Here's how the part is built. I have some questions about the finished solid (model axes, mm). Face numbers are marked on the shaded views. A direction names the side the tool comes from. Round coordinates to 2 decimals unless told otherwise and drop trailing zeros. Loops run counter-clockwise (first coordinate to the right, second up) from the corner with the lowest first, then second, coordinate; pieces in that order, holes last. Notation, with made-up numbers: M 0,85.5 L 42,85.5 A24 ccw 42,107.5 Z; hole C 38.25,-17 d2. An arc over 180 degrees is marked long. Answer as a JSON object with one key per item and string values.
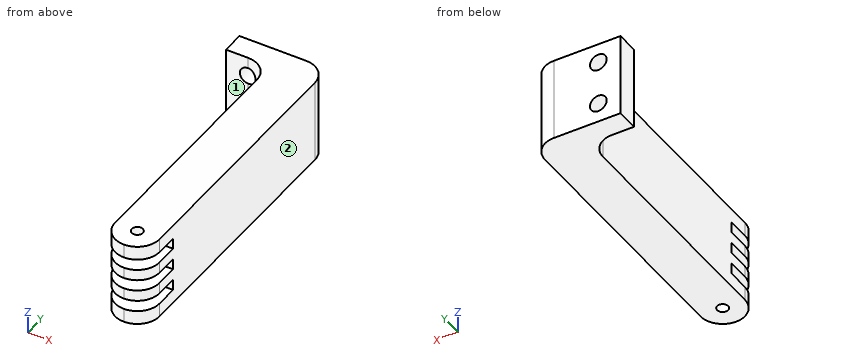
Autodesk Inventor part; units mm, degrees
ref_plane "YZ Plane" through (0, 0, 0) normal (1, 0, 0) x (0, 1, 0)
ref_plane "XZ Plane" through (0, 0, 0) normal (0, 1, 0) x (-1, 0, 0)
ref_plane "XY Plane" through (0, 0, 0) normal (0, 0, 1) x (1, 0, 0)
sketch "Sketch1" plane through (0, 0, 0) normal (0, 0, 1) x (1, 0, 0)
  line L0 (0, 0) -> (0, 50)
  line L1 (0, 50) -> (-8, 50)
  line L2 (0, 0) -> (8, 0)
  line L3 (8, 0) -> (8, 54)
  line L4 (8, 54) -> (-8, 54)
  line L5 (8, 54) -> (-8, 54)
  line L6 (-8, 54) -> (-8, 50)
  dimension "d0" = 50
  dimension "d3" = 8
  dimension "d7" = 54
  dimension "d28" = 16
extrude "Extrusion1" add sketch "Sketch1" along normal blind 15
sketch "Sketch2" plane through (-8, 54, 0) normal (0, 1, 0) x (1, 0, 0)
  line L0 (16, 0) -> (0, 0) construction
  line L1 (1.2766, 0) -> (1.2766, -15) construction
  line L2 (16, -15) -> (0, -15) construction
  line L3 (1.2766, 0) -> (1.2766, -2.75) construction
  line L4 (1.2766, -15) -> (1.2766, -12.25) construction
  line L5 (1.2766, 0) -> (1.2766, -3.5) construction
  line L6 (1.2766, -15) -> (1.2766, -11.5) construction
  line L7 (8, 0) -> (0, 0) construction
  line L8 (0, 0) -> (0, -15) construction
  line L9 (4, 0) -> (4, -15) construction
  line L10 (4, -15) -> (4, -11.5) construction
  line L11 (4, 0) -> (4, -3.5) construction
  circle A0 centre (4, -3.5) radius 1.5
  circle A1 centre (4, -11.5) radius 1.5
  dimension "d12" = 3.5
  dimension "d13" = 3.5
  dimension "d29" = 3.5
  dimension "d30" = 3.5
  dimension "d31" = 3
  dimension "d32" = 3
extrude "Extrusion2" cut sketch "Sketch2" against normal blind 8.75
sketch "Sketch3" plane through (8, 0, 0) normal (1, 0, 0) x (0, 0, -1)
  line L0 (0, 0) -> (-15, 0) construction
  line L1 (-7.5, 0) -> (-7.5, 8) construction
  line L2 (-7.5, 8) -> (-6.5, 8)
  line L3 (-6.5, 8) -> (-8.5, 8)
  line L4 (-8.5, 8) -> (-8.5, 0)
  line L5 (-6.5, 8) -> (-6.5, 0)
  line L6 (-6.5, 0) -> (-4.5, 0)
  line L7 (-4.5, 0) -> (-4.5, 8)
  line L8 (-4.5, 8) -> (-2.5, 8)
  line L9 (-2.5, 8) -> (-2.5, 0)
  line L10 (-8.5, 0) -> (-10.5, 0)
  line L11 (-10.5, 0) -> (-10.5, 8)
  line L12 (-10.5, 8) -> (-12.5, 8)
  line L13 (-12.5, 8) -> (-12.5, 0)
  line L14 (-2.5, 0) -> (0, 0)
  line L15 (-12.5, 0) -> (-15, 0)
  line L16 (-15, 0) -> (-15, 10)
  line L17 (-15, 50) -> (-15, 0)
  line L18 (-15, 10) -> (0, 10)
  line L19 (0, 50) -> (0, 0)
  line L20 (0, 0) -> (0, 10)
  line L21 (-15, 0) -> (0, 0)
  dimension "d18" = 8
  dimension "d19" = 1
  dimension "d20" = 2
  dimension "d21" = 2
  dimension "d22" = 2
  dimension "d23" = 2
  dimension "d24" = 2
  dimension "d25" = 10
extrude "Extrusion3" cut sketch "Sketch3" against normal blind 10.25 contours L2 L5 L21 L4 L3 | L7 L8 L9 L21 | L21 L13 L12 L11
fillet "Fillet1" radius 4 8 edges at (8, 0, 1.25) (8, 0, 5.5) (8, 0, 9.5) (8, 0, 13.75) (0, 0, 13.75) (0, 0, 9.5) (0, 0, 5.5) (0, 0, 1.25)
sketch "Sketch4" plane through (0, 0, 15) normal (0, 0, 1) x (1, 0, 0)
  line L0 (0, 4) -> (8, 4) construction
  circle A0 centre (4, 4) radius 1
  point P0 (0, 0)
  dimension "d34" = 2
extrude "Extrusion4" cut sketch "Sketch4" against normal blind 21
fillet "Fillet2" radius 4 2 edges at (8, 54, 7.5) (0, 50, 7.5)
properties part number "WebcamArm"
Item 1: For P1, Ø1.6, axis at x = 5.5, z = 3.5, coming from the -Y side; P2, Ø2, axis at x = -6, z = 9, coming from the -Y side; P3, Ø7.5, axis at y = 22.5, z = 4, coming from the -X side, each with a flat end and sliding along its axis, tell me the tip position at first contact or that it passes through.
Solution:
{"P1": "stops at y = 8", "P2": "stops at y = 50", "P3": "stops at x = 0"}
Item 2: I want a section at D-D on y = 26. List the corners of the cut face in (x, z) for me.
Solution:
{"outline": "M 0,0 L 8,0 L 8,15 L 0,15 Z"}
Item 3: If I drill on L1, parallel to Z at x = -4, y = 53.05; L2, parallel to Y at x = 4, z = 13.55; L3, parallel to Y at x = -6.75, z = 1.5, over which ranges is the centre line in solid material (lowest first)? Write a range as from..to.
Solution:
{"L1": "z = 0..2, 5..10, 13..15", "L2": "y = 0..3, 5..54", "L3": "y = 50..54"}
Item 4: I want a section at A-A on z = 3.5. List the corners of the cut face in (x, y) for me.
Solution:
{"outline": "M -8,50 L -5.5,50 L -5.5,54 L -8,54 Z; M -2.5,49.71 A4 cw 0,46 L 0,8 L 8,8 L 8,50 A4 ccw 4,54 L -2.5,54 Z"}
Item 5: I want a section at C-C on x = 5.75. List the corners of the cut face in (y, z) for me.
Solution:
{"outline": "M 0.4,0 L 53.6,0 L 53.6,15 L 0.4,15 L 0.4,12.5 L 8,12.5 L 8,10.5 L 0.4,10.5 L 0.4,8.5 L 8,8.5 L 8,6.5 L 0.4,6.5 L 0.4,4.5 L 8,4.5 L 8,2.5 L 0.4,2.5 Z"}
Item 6: For the marked faces 1 and 2, which set-ups out of +Z, -Z, +X, -X, +Y, -Y let a thin tool reach every point of the face, with its end or its side?
Solution:
{"face 1": "+Z, -Z, -X, -Y", "face 2": "+Z, -Z, +X, +Y, -Y"}
